```python
from build123d import *

# Parameters (mm, degrees)
F0_R     = 7.198052
F0_R_2   = 6.829302
F1_DEPTH = 50.8
F2_R     = 12.108845
F3_DEPTH = 127
F4_W     = 2.642531
F4_H     = 6.459523
F4_W_2   = 2.348915
F4_H_2   = 7.340368
F5_DEPTH = 50.8
F6_W     = 3.81699
F6_H     = 8.221211
F6_W_2   = 4.404219
F6_W_3   = 4.110609
F6_W_4   = 3.523376
F7_DEPTH = 101.6


with BuildPart() as f1:
    # F0 (on Front) → F1 (new body)
    with BuildSketch(Plane.XZ):
        with BuildLine():
            Line((68.852641, 38.757138), (45.363467, 38.757138))
            Line((45.363467, 38.757138), (0, 27.155228))
            Line((0, 27.155228), (-69.439873, 9.39567))
            Line((-69.439873, 9.39567), (-88.524826, -12.919046))
            Line((-88.524826, -12.919046), (92.63543, -12.919046))
            ThreePointArc((92.63543, -12.919046), (101.629006, 17.76077), (77.51909, 38.757138))
            Line((77.51909, 38.757138), (68.852641, 38.757138))
        make_face()
        with Locations((-54.171909, -4.697835)):
            Circle(F0_R, mode=Mode.SUBTRACT)
        with Locations((65.329269, -4.697835)):
            Circle(F0_R_2, mode=Mode.SUBTRACT)
        with BuildLine():
            ThreePointArc((77.51909, 38.757138), (73.185865, 39.07565), (68.852641, 38.757138))
            Line((68.852641, 38.757138), (77.51909, 38.757138))
        make_face()
    extrude(amount=F1_DEPTH)

    # F2 (on Right) → F3 (cut)
    with BuildSketch(Plane.YZ):
        with Locations((-24.810441, 14.680734)):
            Circle(F2_R)
    extrude(amount=F3_DEPTH, mode=Mode.SUBTRACT)

    # F4 (on Front) → F5 (join)
    with BuildSketch(Plane.XZ):
        Polygon((48.69454, 52.263413), (48.69454, 44.042204), (56.622133, 44.042204), (59.264664, 44.042204), (69.247566, 44.042204), (71.596481, 44.042204), (80.992155, 44.042204), (102.719635, 62.83354), (88.332519, 62.83354), align=None)
        with Locations((57.943399, 40.812443)):
            Rectangle(F4_W, F4_H)
        with Locations((70.422023, 40.37202)):
            Rectangle(F4_W_2, F4_H_2)
    extrude(amount=F5_DEPTH)

    # F6 (on Right) → F7 (cut)
    with BuildSketch(Plane.YZ):
        with Locations((-9.982899, -1.468074)):
            Rectangle(F6_W, F6_H)
        with Locations((-21.433872, -1.468074)):
            Rectangle(F6_W_2, F6_H)
        with Locations((-33.618881, -1.468074)):
            Rectangle(F6_W_3, F6_H)
        with Locations((-43.308167, -1.468074)):
            Rectangle(F6_W_4, F6_H)
    extrude(amount=-F7_DEPTH, mode=Mode.SUBTRACT)


solid = f1.part
```
CAD build for the part. Positions are in the model's coordinates, mm. A direction names the side the tool comes from. Coordinates: 2 decimals unless noted, no trailing zeros. Loops run counter-clockwise (first coordinate to the right, second up) from the corner with the lowest first, then second, coordinate; pieces in that order, holes last. Notation, with made-up numbers: (17, 16) - (70, 16) arc R21 cw to (70, 36) - close; hole circle Ø7 at (73.5, -29.75). An arc over 180 degrees is marked (long way). Return JSON: item names as keys, results as strings.
1. Band-saw the part on D-D (y = -2.5). Give the cut face in (x, z), and give its area (3 significant figures).
Result:
{"outline": "(-88.52, -12.92) - (92.64, -12.92) arc R29.64 ccw to (77.52, 38.76) arc R29.64 ccw to (71.6, 39.03) - (71.6, 44.04) - (80.99, 44.04) - (102.72, 62.83) - (88.33, 62.83) - (48.69, 52.26) - (48.69, 44.04) - (56.62, 44.04) - (56.62, 38.76) - (45.36, 38.76) - (-69.44, 9.4) - close; hole circle Ø14.4 at (-54.17, -4.7); hole circle Ø13.66 at (65.33, -4.7); hole (59.26, 38.76) - (68.85, 38.76) arc R29.64 cw to (69.25, 38.81) - (69.25, 44.04) - (59.26, 44.04) - close", "area": "7,500 mm2"}
2. Drop flat-ended pins along their axis: pin 1 (9 mm diameter, centred on x = 52, y = -29, fed in from +Z); pin 2 (1.5 mm diameter, centred on x = -43.5, y = -10.5, fed in from +Z); pin 3 (3 mm diameter, centred on y = -13, z = 32.5, fed in from +X). Give the stop position or say it passes through.
Result:
{"pin 1": "stops at z = 54.34", "pin 2": "stops at z = 16.22", "pin 3": "stops at x = 93.52"}
3. 3-axis set-ups, long thin cutter, end or side, ignore diameter. For faces 1 (the flat face through (51, -25, 38.757)), 2 (the flat face through (69.248, -25, 41)), 3 (the flat face through (91.704, -25.044, 53.306)), 4 (the flat face through (-41, -41.546, -2)), 5 (the cylindrical face through (50.69, -27.44, 2.86)): which of +Z, -Z, +X, -X, +Y, -Y reach the whole face in a straight line?
Result:
{"face 1": "-X, +Y, -Y", "face 2": "+Y, -Y", "face 3": "+X, +Y, -Y", "face 4": "-X", "face 5": "+X"}
4. Probe L1, parallel to Z at x = 75, y = -24.5; L2, parallel to X at y = -41, z = 44; L3, parallel to X at y = -39, z = -10. List the from-to ranges inside material, lowest first. Write a range as from..to.
Result:
{"L1": "z = -12.92..2.58, 26.79..39.02, 44.04..59.28", "L2": "x = 56.62..59.26, 69.25..71.6", "L3": "x = -86.03..-59.04, -49.3..61.03, 69.63..95.55"}
5. Mould opens along Y. For faces 6 (the flat face through (-41, -35.674, -2)), 7 (the flat face through (0, -34, -1)), 8 (the flat face through (68.791, -25.044, 57.622)) say: released by +Y, released by -Y, zero draft, split by the parting line, or undercut.
Result:
{"face 6": "undercut", "face 7": "undercut", "face 8": "zero draft"}
6. Band-saw the part on A-A (y = -27.5). Give the cut face in (x, z), and give its area (3 significant figures).
Result:
{"outline": "(-88.52, -12.92) - (92.64, -12.92) arc R29.64 ccw to (102.08, 2.87) - (0, 2.87) - (0, 26.49) - (97.43, 26.49) arc R29.64 ccw to (77.52, 38.76) arc R29.64 ccw to (71.6, 39.03) - (71.6, 44.04) - (80.99, 44.04) - (102.72, 62.83) - (88.33, 62.83) - (48.69, 52.26) - (48.69, 44.04) - (56.62, 44.04) - (56.62, 38.76) - (45.36, 38.76) - (-69.44, 9.4) - close; hole circle Ø14.4 at (-54.17, -4.7); hole circle Ø13.66 at (65.33, -4.7); hole (59.26, 38.76) - (68.85, 38.76) arc R29.64 cw to (69.25, 38.81) - (69.25, 44.04) - (59.26, 44.04) - close", "area": "5,100 mm2"}
7. Band-saw the part on B-B (x = -14.5). Give the cut face in (y, z).
Result:
{"outline": "(-50.8, -12.92) - (0, -12.92) - (0, 23.45) - (-50.8, 23.45) - close; hole (-45.07, -5.58) - (-41.55, -5.58) - (-41.55, 2.64) - (-45.07, 2.64) - close; hole (-35.67, -5.58) - (-31.56, -5.58) - (-31.56, 2.64) - (-35.67, 2.64) - close; hole (-23.64, -5.58) - (-19.23, -5.58) - (-19.23, 2.64) - (-23.64, 2.64) - close; hole (-11.89, -5.58) - (-8.07, -5.58) - (-8.07, 2.64) - (-11.89, 2.64) - close"}
8. Band-saw the part on C-C (z = 6). Give the cut face in (x, y).
Result:
{"outline": "(-72.34, -50.8) - (102.62, -50.8) - (102.62, -33.25) - (0, -33.25) - (0, -16.37) - (102.62, -16.37) - (102.62, 0) - (-72.34, 0) - close"}
